```python
from build123d import *

# Parameters (mm, degrees)
SKETCH1_R           = 23.525
SKETCH1_R_2         = 1.5
BOSS_EXTRUDE1_DEPTH = 10


with BuildPart() as part:
    # Sketch1 → Boss-Extrude1 (new body)
    with BuildSketch(Plane.XY):
        with BuildLine():
            Line((0, -35), (-129, -35))
            ThreePointArc((-129, -35), (-142.388025128, -32.338224799), (-153.739712354, -24.757759039))
            Line((-153.739712354, -24.757759039), (-189.107939553, 10.584687182))
            Line((-189.107939553, 10.584687182), (-182.180820093, 17.516859712))
            Line((-182.180820093, 17.516859712), (-189.112992624, 24.443979172))
            Line((-189.112992624, 24.443979172), (-184.165050154, 29.395530979))
            Line((-184.165050154, 29.395530979), (-187.701872873, 32.929775601))
            Line((-187.701872873, 32.929775601), (-178.230097286, 42.408460491))
            Line((-178.230097286, 42.408460491), (-174.693274566, 38.874215869))
            Line((-174.693274566, 38.874215869), (-167.907524892, 45.664915491))
            Line((-167.907524892, 45.664915491), (-171.444347612, 49.199160113))
            Line((-171.444347612, 49.199160113), (-161.972572025, 58.677845002))
            Line((-161.972572025, 58.677845002), (-158.435749305, 55.14360038))
            Line((-158.435749305, 55.14360038), (-153.487806834, 60.095152188))
            Line((-153.487806834, 60.095152188), (-146.555634303, 53.168032728))
            Line((-146.555634303, 53.168032728), (-139.628514844, 60.100205259))
            Line((-139.628514844, 60.100205259), (-117.439262294, 37.927127131))
            ThreePointArc((-117.439262294, 37.927127131), (-114.195654931, 35.760716243), (-110.37, 35))
            Line((-110.37, 35), (0, 35))
            ThreePointArc((0, 35), (35, 0), (0, -35))
        make_face()
        Circle(SKETCH1_R, mode=Mode.SUBTRACT)
        with Locations((29, 0)):
            Circle(SKETCH1_R_2, mode=Mode.SUBTRACT)
        with Locations((0, 29)):
            Circle(SKETCH1_R_2, mode=Mode.SUBTRACT)
        with Locations((0, -29)):
            Circle(SKETCH1_R_2, mode=Mode.SUBTRACT)
        with Locations((-50, -29)):
            Circle(SKETCH1_R_2, mode=Mode.SUBTRACT)
        with Locations((-50, 29)):
            Circle(SKETCH1_R_2, mode=Mode.SUBTRACT)
        with Locations((-100, -29)):
            Circle(SKETCH1_R_2, mode=Mode.SUBTRACT)
        with Locations((-100, 29)):
            Circle(SKETCH1_R_2, mode=Mode.SUBTRACT)
        with Locations((-29, 0)):
            Circle(SKETCH1_R_2, mode=Mode.SUBTRACT)
        with Locations((-169.166963878, 9.036324012)):
            Circle(SKETCH1_R_2, mode=Mode.SUBTRACT)
        with Locations((-138.065609793, 40.160362537)):
            Circle(SKETCH1_R_2, mode=Mode.SUBTRACT)
        with Locations((-138.576564013, -26.311393382)):
            Circle(SKETCH1_R_2, mode=Mode.SUBTRACT)
        with BuildLine():
            Line((-58, -5), (-61, -5))
            ThreePointArc((-61, -5), (-66, 0), (-61, 5))
            Line((-61, 5), (-58, 5))
            ThreePointArc((-58, 5), (-53, 0), (-58, -5))
        make_face(mode=Mode.SUBTRACT)
        with BuildLine():
            Line((-58, 16), (-61, 16))
            ThreePointArc((-61, 16), (-63.5, 18.5), (-61, 21))
            Line((-61, 21), (-58, 21))
            ThreePointArc((-58, 21), (-55.5, 18.5), (-58, 16))
        make_face(mode=Mode.SUBTRACT)
        with BuildLine():
            Line((-58, -21), (-61, -21))
            ThreePointArc((-61, -21), (-63.5, -18.5), (-61, -16))
            Line((-61, -16), (-58, -16))
            ThreePointArc((-58, -16), (-55.5, -18.5), (-58, -21))
        make_face(mode=Mode.SUBTRACT)
        Polygon((-173.557263216, 26.146707149), (-155.179191181, 44.538185292), (-148.108123369, 37.46711748), (-166.492898458, 19.082342391), align=None, mode=Mode.SUBTRACT)
    extrude(amount=BOSS_EXTRUDE1_DEPTH)


solid = part.part
```
Geometry check sheet. Reference: the model listing, model coordinates, mm. A direction names the side the tool comes from. Round coordinates to 2 decimals unless told otherwise and drop trailing zeros. Loops run counter-clockwise (first coordinate to the right, second up) from the corner with the lowest first, then second, coordinate; pieces in that order, holes last. Notation, with made-up numbers: (63, 60) - (116, 60) arc R7 ccw to (116, 68) - close; hole circle Ø1 at (-3.5, 48.5). An arc over 180 degrees is marked (long way). Write each question's results on one line, items separated by ' | '. Start each with the question number.
Q1. Thickness scan on line 1 (Y direction, x = -50, z = 7.75); line 2 (Y direction, x = -1, z = 5); line 3 (Y direction, x = -168, z = 9.5). Record the ranges inside material, lowest first. Write a range as [from, to].
Q2. Release check for a two-part mould opening along X. For faces 6 (the flat face through (-169.98, 22.57, 4.93)), 7 (the cylindrical face through (-142.21, -32.41, 4.93)), 8 (the flat face through (-171.35, 42.22, 4.93)), 9 (the cylindrical face through (-114.246, 35.782, 4.93)) record: +X half, -X half, draft (parallel to the pull), parting line (faces both ways), or undercut.
Q3. Cross-section at B-B on x = -104. Enter the section's corners in (y, z).
Q4. Access from +Z, -Z, +X, -X, +Y, -Y to the whole of each face (thin tool, end or side, straight path). Record for faces 1 (the flat face through (-156, 57.58, 4.93)), 2 (the flat face through (-171.18, -7.33, 4.93)), 3 (the cylindrical face through (-53, 0, 5)), 4 (the flat face through (-128.69, 49.17, 4.93)), 5 (the flat face through (-185.598, 20.932, 4.93)).
Q5. Cross-section at A-A on y = -12.5. Enter the section's corners in (x, z).
Q6. Cross-section at C-C on z = 2.25. State how many separate pieces and enclosed holes the cut face has, and give its area (3 significant figures).
Q7. Gauge pin test, flat ends, axial feed: P1, Ø1.8, axis at x = -29, y = 0, coming from the -Z side; P2, Ø3, axis at y = 47.5, z = 3.5, coming from the +X side; P3, Ø6, axis at y = -14.5, z = 3, coming from the +X side; P4, Ø1.5, axis at x = -60, z = 4.5, coming from the +Y side. Record the tip position at first contact, or that the pin passes through.
Answers below:
1) line 1: y = [-35, -30.5], [-27.5, 27.5], [30.5, 35] | line 2: y = [-35, -30.12], [-27.88, -23.5], [23.5, 27.88], [30.12, 35] | line 3: y = [-10.51, 8.09], [9.98, 20.59], [31.71, 45.57], [45.76, 52.65]
2) face 6: undercut | face 7: -X half | face 8: undercut | face 9: +X half
3) outline: (-35, 0) - (35, 0) - (35, 10) - (-35, 10) - close
4) face 1: +Z, -Z, +Y | face 2: +Z, -Z, -X, -Y | face 3: +Z, -Z | face 4: +Z, -Z, +X, +Y | face 5: +Z, -Z, -X
5) outline: (-166.01, 0) - (-19.93, 0) - (-19.93, 10) - (-166.01, 10) - close; (19.93, 0) - (32.69, 0) - (32.69, 10) - (19.93, 10) - close
6) separate pieces: 1 | enclosed holes: 16 | area: 12,800 mm²
7) P1: passes through | P2: stops at x = -125.52 | P3: stops at x = 33.06 | P4: stops at y = 35
